Read the model definition and answer for the solid it produces. Units are mm, in the model's axes. Coordinates: 2 decimals unless noted, no trailing zeros. Loops run counter-clockwise (first coordinate to the right, second up) from the corner with the lowest first, then second, coordinate; pieces in that order, holes last. Notation, with made-up numbers: (-11.5, 58) -> (8.5, 58) arc R14 ccw to (8.5, 80) -> close; hole circle Ø6 at (23, -3.5). An arc over 180 degrees is marked (long way). Answer as a JSON object with one key per item and string values. Group by question number.
1) Consider probe 1 along Z at (x, y) = (34, -15.75); probe 2 along X at (y, z) = (-2.75, 34.5); probe 3 along X at (y, z) = (-10.75, 31.5). Determine where each line is inside the solid, lowest interval first. Write a range as [from, to].
2) Section A-A, the plane y = -8.5 is taken. Give the vertices of the cut face in (x, z).
3) Flat-ended cylindrical pins translate along their axes: P1, Ø8, axis at x = 18.5, z = 5, coming from the +Y side; P2, Ø2, axis at x = 31, y = -6, coming from the +Z side; P3, Ø1, axis at y = -2.5, z = 20.5, coming from the +X side. Find the tip coordinate at first contact, or state that the pin passes through.
4) Section C-C, the plane x = 23.5 is taken. Give the vertices of the cut face in (y, z), plus the area to 3 significant figures.
5) Section B-B, the plane z = 30.5 is taken. Give the vertices of the cut face in (x, y), plus the area to 3 significant figures.
from build123d import *

# Parameters (mm, degrees)
F0_W     = 57.15
F0_H     = 38.1
F1_DEPTH = 25.4
F3_DEPTH = 25.4
F4_R     = 5.08


with BuildPart() as f1:
    # F0 (on Front) → F1 (new body)
    with BuildSketch(Plane.XZ):
        with Locations((11.729645, 19.05)):
            Rectangle(F0_W, F0_H)
    extrude(amount=F1_DEPTH)

    # F2 (on face) → F3 (cut)
    with BuildSketch(Plane.XZ.offset(25.4)):
        with BuildLine():
            Line((40.304645, 38.1), (21.254645, 38.1))
            ThreePointArc((21.254645, 38.1), (28.622933, 26.418288), (40.304645, 19.05))
            Line((40.304645, 19.05), (40.304645, 38.1))
        make_face()
    extrude(amount=-F3_DEPTH, mode=Mode.SUBTRACT)

    # F4
    f4_edges = [f1.edges().sort_by_distance(p)[0] for p in [
        (-16.845355, -12.7, 38.1),
    ]]
    fillet(f4_edges, radius=F4_R)


solid = f1.part
Determined:
{
 "1": {"probe 1": "[0, 22.11]", "probe 2": "[-16.62, 22.79]", "probe 3": "[-16.85, 24.51]"},
 "2": {"outline": "(-16.85, 0) -> (40.3, 0) -> (40.3, 19.05) arc R31.27 cw to (21.25, 38.1) -> (-11.77, 38.1) arc R5.08 ccw to (-16.85, 33.02) -> close"},
 "3": {"P1": "y = 0", "P2": "z = 25.12", "P3": "x = 37.93"},
 "4": {"outline": "(-25.4, 0) -> (0, 0) -> (0, 33.16) -> (-25.4, 33.16) -> close", "area": "842 mm²"},
 "5": {"outline": "(-16.85, -25.4) -> (25.19, -25.4) -> (25.19, 0) -> (-16.85, 0) -> close", "area": "1,070 mm²"}
}
